from build123d import *

# Parameters (mm, degrees)
EXTRUDE_1_DEPTH             = 3
EXTRUDE_2_DEPTH             = 14
CUT_EXTRUDE_1_REACH         = 66.954
SKETCH_5_W                  = 36
SKETCH_5_H                  = 13
HOLE_WIZARD_3_0_3_1_D       = 3
HOLE_WIZARD_3_0_3_1_DEPTH   = 3
HOLE_WIZARD_3_0_3_1_TIP     = 0.901290929
HOLE_WIZARD_3_2_3_2_1_D     = 3.2
HOLE_WIZARD_3_2_3_2_1_DEPTH = 17
HOLE_WIZARD_3_2_3_2_2_D     = 3.2
CHAMFER_1_SIZE              = 1.55
FILLET_1_R                  = 1
FILLET_2_R                  = 3
FILLET_3_R                  = 4


with BuildPart() as part:
    # Эскиз1 → Бобышка-Вытянуть1 (new body)
    with BuildSketch(Plane(origin=(0, 17, 0), x_dir=(1, 0, 0), z_dir=(0, 1, 0))):
        with BuildLine():
            Line((23, 30.854497241), (23, 27.694764848))
            ThreePointArc((23, 27.694764848), (0, 36), (-23, 27.694764848))
            Line((-23, 27.694764848), (-23, 30.854497241))
            ThreePointArc((-23, 30.854497241), (-25.347212259, 34.497064012), (-29.634146341, 33.864692094))
            ThreePointArc((-29.634146341, 33.864692094), (0, -45), (29.634146341, 33.864692094))
            ThreePointArc((29.634146341, 33.864692094), (25.347212259, 34.497064012), (23, 30.854497241))
        make_face()
    extrude(amount=-EXTRUDE_1_DEPTH)

    # Эскиз2 → Бобышка-Вытянуть2 (add)
    with BuildSketch(Plane.XZ.offset(-14)):
        with BuildLine():
            Line((-23, -27.694764848), (-23, -30.248966925))
            ThreePointArc((-23, -30.248966925), (-12.293870341, 35.956372899), (36.705181399, -9.835123714))
            Line((36.705181399, -9.835123714), (43.466662183, -11.64685703))
            ThreePointArc((43.466662183, -11.64685703), (41.574578963, -17.220754456), (38.97114317, -22.5))
            Line((38.97114317, -22.5), (32.908965344, -19))
            ThreePointArc((32.908965344, -19), (28.514696486, -25.117963379), (23, -30.248966925))
            Line((23, -30.248966925), (23, -27.694764848))
            ThreePointArc((23, -27.694764848), (0, -36), (-23, -27.694764848))
        make_face()
    extrude(amount=EXTRUDE_2_DEPTH)

    # Эскиз4 → Вырез-Вытянуть1 (cut, up to next)
    with BuildSketch(Plane(origin=(0, 4, 0), x_dir=(1, 0, 0), z_dir=(0, 1, 0)), mode=Mode.PRIVATE) as cut_extrude_1_sk1:
        with BuildLine():
            Line((-23, 27.694764848), (-23, 20))
            Line((-23, 20), (23, 20))
            Line((23, 20), (23, 27.694764848))
            ThreePointArc((23, 27.694764848), (0, 36), (-23, 27.694764848))
        make_face()
    cut_extrude_1_tool1 = extrude(cut_extrude_1_sk1.sketch, amount=-CUT_EXTRUDE_1_REACH, mode=Mode.PRIVATE) & part.part
    add(cut_extrude_1_tool1.solids().sort_by_distance((0, 4, -26.906646))[0], mode=Mode.SUBTRACT)

    # Эскиз5 → Вырез-Повернуть1 (revolve, cut)
    with BuildSketch(Plane(origin=(0, 0, 0), x_dir=(-1, 0, 0), z_dir=(0, 0, -1))):
        with Locations((-18, 10.5)):
            Rectangle(SKETCH_5_W, SKETCH_5_H)
    revolve(axis=Axis((0, 4, 0), (0, 1, 0)), mode=Mode.SUBTRACT)

    # Диаметр отверстия Ø3.0 (3)1
    with Locations(Plane(origin=(0, 0, 0), x_dir=(-1, 0, 0), z_dir=(0, -1, 0))):
        with Locations((0, -12.5), (0, 12.5)):
            Hole(HOLE_WIZARD_3_0_3_1_D / 2, depth=HOLE_WIZARD_3_0_3_1_DEPTH)
            with Locations((0, 0, -(HOLE_WIZARD_3_0_3_1_DEPTH + HOLE_WIZARD_3_0_3_1_TIP / 2))):  # 118° drill point
                Cone(0, HOLE_WIZARD_3_0_3_1_D / 2, HOLE_WIZARD_3_0_3_1_TIP, mode=Mode.SUBTRACT)

    # Диаметр отверстия Ø3.2 (3.2)1
    with Locations(Plane(origin=(0, 17, 0), x_dir=(1, 0, 0), z_dir=(0, 1, 0))):
        with Locations((29.344931419, -29.344931419), (0, -41.5), (-29.344931419, -29.344931419), (-41.5, 0), (-29.344931419, 29.344931419), (29.344931419, 29.344931419), (41.5, 0)):
            Hole(HOLE_WIZARD_3_2_3_2_1_D / 2, depth=HOLE_WIZARD_3_2_3_2_1_DEPTH)

    # Диаметр отверстия Ø3.2 (3.2)2 (through all)
    with Locations(Plane(origin=(0, 4, 0), x_dir=(1, 0, 0), z_dir=(0, 1, 0))):
        with Locations((-6.25, -10.825317547), (6.25, -10.825317547), (12.5, 0), (6.25, 10.825317547), (-6.25, 10.825317547), (-12.5, 0)):
            Hole(HOLE_WIZARD_3_2_3_2_2_D / 2)

    # Фаска1
    chamfer_1_edges = [part.edges().sort_by_distance(p)[0] for p in [
        (-10.9, 4, 0),
        (-4.65, 4, -10.825317547),
        (7.85, 4, -10.825317547),
        (14.1, 4, 0),
        (7.85, 4, 10.825317547),
        (-4.65, 4, 10.825317547),
    ]]
    chamfer(chamfer_1_edges, length=CHAMFER_1_SIZE)

    # Скругление1
    # the kernel refuses this fillet: 1 mm, written as the material it takes off along each edge
    with BuildSketch(Plane(origin=(38.97114317, 14, -22.5), x_dir=(-0.8660254037844388, 0, 0.4999999999999999), z_dir=(0, -1, 0))) as fillet_1_piece_1:
        with BuildLine():
            CenterArc((1.011365104, -1), FILLET_1_R, 90, 91.302288935)
            ThreePointArc((0.011623402, -1.022727273), (0.002905944, -0.511396661), (0, 0))
            Line((0, 0), (1.011365104, 0))
        make_face()
    extrude(amount=16.556983303, mode=Mode.SUBTRACT)
    with BuildSketch(Plane(origin=(43.466662183, 14, -11.64685703), x_dir=(-0.9659258262890692, 0, 0.2588190451025174), z_dir=(0, -1, 0))) as fillet_1_piece_2:
        with BuildLine():
            CenterArc((1.011365104, 1), FILLET_1_R, 178.697711065, 91.302288935)
            ThreePointArc((0.011623402, 1.022727273), (0.002905944, 0.511396661), (0, 0))
            Line((0, 0), (1.011365104, 0))
        make_face()
    extrude(amount=16.556983303, mode=Mode.SUBTRACT)

    # Скругление2
    fillet_2_edges = [part.edges().sort_by_distance(p)[0] for p in [
        (32.908965344, 7, -19),
        (36.705181399, 7, -9.835123714),
    ]]
    fillet(fillet_2_edges, radius=FILLET_2_R)

    # Скругление3
    fillet_3_edges = [part.edges().sort_by_distance(p)[0] for p in [
        (23, 10.5, -27.694764848),
        (-23, 10.5, -27.694764848),
        (-23, 2, -20),
        (23, 2, -20),
    ]]
    fillet(fillet_3_edges, radius=FILLET_3_R)


with BuildPart() as body_2:
    # Зеркальное отражение1: mirrored copy
    add(part.part.mirror(Plane(origin=(27, 17, -30.854497241), x_dir=(0, 0, 1), z_dir=(0, 1, 0))))


solid = body_2.part
Design review of the part built by this model. Coordinates are the model's own, in mm. A direction names the side the tool comes from. Round coordinates to 2 decimals unless told otherwise and drop trailing zeros. Loops run counter-clockwise (first coordinate to the right, second up) from the corner with the lowest first, then second, coordinate; pieces in that order, holes last. Notation, with made-up numbers: M 13.25,1 L 34.25,1 A23 cw 34.25,10 Z; hole C -12.75,-11.5 d11. An arc over 180 degrees is marked long. Answer as a JSON object with one key per item and string values.
Item 1: Machinability: for faces 1 (the cylindrical face through (4.724, 32.792, 10.345)), 2 (the cylindrical face through (23.35, 23.59, -27.88)), 3 (the cylindrical face through (0, 32, 14)), 4 (the cylindrical face through (21.797, 32.028, -21.141)), which of the approach directions +Z, -Z, +X, -X, +Y, -Y give a long, thin tool a straight path to every point of the face, cutting with its end or side? Answer none if there is none.
Answer sheet:
{"face 1": "+Y, -Y", "face 2": "-Y", "face 3": "+Y", "face 4": "-Z, +Y, -Y"}
Item 2: The part is to be moulded in two halves that separate along X. For faces 5 (the conical face through (-0.12, 30.255, -12.269)), 6 (the cylindrical face through (-14.652, 26.902, 35.062)), say which applies: pulls with the +X half, pulls with the -X half, needs draft (parallel to the pull), parting line crosses it, or undercut.
Answer sheet:
{"face 5": "undercut", "face 6": "parting line crosses it"}
Item 3: We need section B-B on x = 41.5. Give the boundary of the cut face in (y, z), and give its area (3 significant figures).
Answer sheet:
{"outline": "M 17,-17.4 L 34,-17.4 L 34,-11.12 L 20,-11.12 L 20,-1.6 L 17,-1.6 Z; M 17,1.6 L 20,1.6 L 20,17.4 L 17,17.4 Z", "area": "183 mm^2"}
Item 4: Wall thickness on L1, parallel to X at y = 33.45, z = 0; L2, parallel to Z at x = 6.25, y = 32.95; L3, parallel to Z at x = -31.5, y = 25.5: over which ranges is each line inside the solid? List them lowest first. Write a range as from..to.
Answer sheet:
{"L1": "x = -38..-14.1, -10.9..10.9, 14.1..38", "L2": "z = -20..-12.43, -9.23..9.23, 12.43..37.48", "L3": "z = -21.25..-17.43, 17.43..21.25"}
Item 5: We need section A-A on z = -25.5. Give the boundary of the cut face in (x, y).
Answer sheet:
{"outline": "M -37.08,17 L -25.41,17 L -25.41,30 L -23,30 L -23,34 L -28.17,34 L -28.17,20 L -37.08,20 Z; M 23,30 L 25.41,30 L 25.41,17 L 37.08,17 L 37.08,20 L 28.17,20 L 28.17,34 L 23,34 Z"}
Item 6: Clearance check with flat-ended pins moving along their axes: P1, Ø2, axis at y = 25.5, z = -29, coming from the +X side; P2, Ø10, axis at y = 31, z = -10, coming from the +X side; P3, Ø7.5, axis at x = 32.5, z = -29, coming from the +Y side. State where each tip first meets the part, or that it passes through.
Answer sheet:
{"P1": "stops at x = 25.69", "P2": "stops at x = 43.23", "P3": "stops at y = 20"}
Item 7: We need section C-C on z = 0. State how many separate pieces and enclosed holes the cut face has, and give its area (3 significant figures).
Answer sheet:
{"separate pieces": "5", "enclosed holes": "0", "area": "348 mm^2"}
Item 8: We need section D-D on x = 6.25. Give the boundary of the cut face in (y, z).
Answer sheet:
{"outline": "M 17,35.45 L 30,35.45 L 30,13.98 L 31.55,12.43 L 34,12.43 L 34,37.48 L 20,37.48 L 20,44.56 L 17,44.56 Z; M 30,-20 L 34,-20 L 34,-12.43 L 31.55,-12.43 L 30,-13.98 Z; M 30,-7.68 L 31.55,-9.23 L 34,-9.23 L 34,9.23 L 31.55,9.23 L 30,7.68 Z"}
